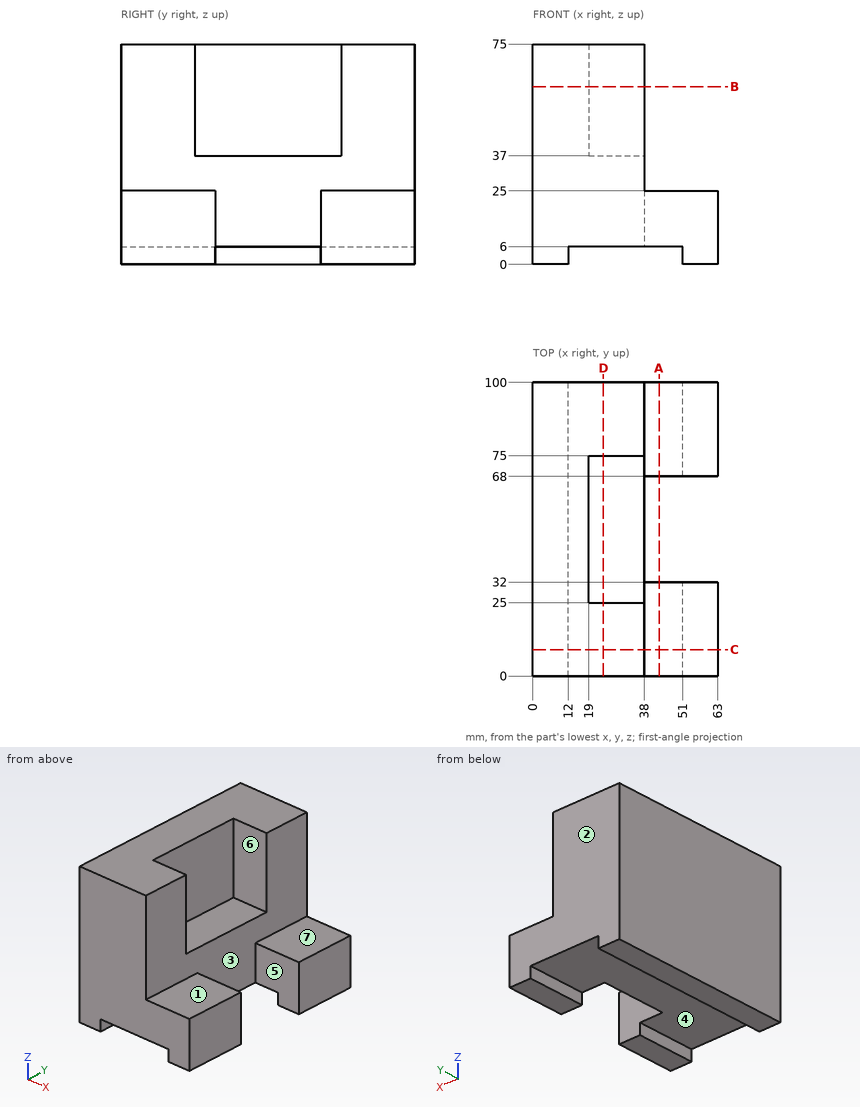
Here's the drawing with two shaded views (mm, measured from the low corner). I have some questions. A direction names the side the tool comes from. Give positions to 0.01 mm unless a question says otherwise; leave off trailing zeros. Loops run counter-clockwise (first coordinate to the right, second up) from the corner with the lowest first, then second, coordinate; pieces in that order, holes last. Notation, with made-up numbers: (82, 2) -> (114, 2) arc R24 cw to (114, 32) -> close; hole circle Ø1 at (48, 42). An arc over 180 degrees is marked (long way). Use one line per item in the form item = value.
1) If we section it at B-B (z = 60.5): Please give me the cut outline in (x, y).
Answers:
outline = (0, 0) -> (38, 0) -> (38, 25) -> (19, 25) -> (19, 75) -> (38, 75) -> (38, 100) -> (0, 100) -> close
2) Will these pins go through, and if not, where does the flat tip stop? pin 1 (9.5 mm diameter, centred on x = 28, z = 63.5, fed in from -Y); pin 2 (4 mm diameter, centred on x = 15.5, y = 86.5, fed in from -Z); pin 3 (19 mm diameter, centred on y = 46, z = 62, fed in from +X); pin 4 (10 mm diameter, centred on x = 41.5, y = 58, fed in from +Z).
Answers:
pin_1 = 0
pin_2 = 6
pin_3 = 19
pin_4 = 37
3) If we section it at A-A (x = 43): Please give me the cut outline in (y, z).
Answers:
outline = (0, 6) -> (32, 6) -> (32, 25) -> (0, 25) -> close; (68, 6) -> (100, 6) -> (100, 25) -> (68, 25) -> close
4) For the marked faces 4, 5, 6 and 7, which set-ups out of +Z, -Z, +X, -X, +Y, -Y let a thin tool reach every point of the face, with its end or its side?
Answers:
face_4 = -Z, +Y, -Y
face_5 = +Z, -Z, +X
face_6 = +Z, +X
face_7 = +Z, +X, +Y, -Y
5) If we section it at D-D (x = 24): Please give me the cut outline in (y, z), plus the area to 3 significant figures.
Answers:
outline = (0, 6) -> (100, 6) -> (100, 75) -> (75, 75) -> (75, 37) -> (25, 37) -> (25, 75) -> (0, 75) -> close
area = 5,000 mm²
6) I need wall thicknesses on line 1 along Y through (x, z) = (32, 59); line 2 along Y through (x, z) = (43, 7.5); line 3 along X through (y, z) = (32, 61). Which ranges of each line are inside material? Lowest first, please.
Answers:
line_1 = 0 to 25, 75 to 100
line_2 = 0 to 32, 68 to 100
line_3 = 0 to 19
7) We'd pull the mould along Y, two halves only. Please class the marked faces 1, 2 and 3: released by +Y, released by -Y, zero draft, split by the parting line, or undercut.
Answers:
face_1 = zero draft
face_2 = released by +Y
face_3 = undercut
8) If we section it at C-C (y = 9): Please give me the cut outline in (x, z), plus the area to 3 significant figures.
Answers:
outline = (0, 0) -> (12, 0) -> (12, 6) -> (51, 6) -> (51, 0) -> (63, 0) -> (63, 25) -> (38, 25) -> (38, 75) -> (0, 75) -> close
area = 3,240 mm²
